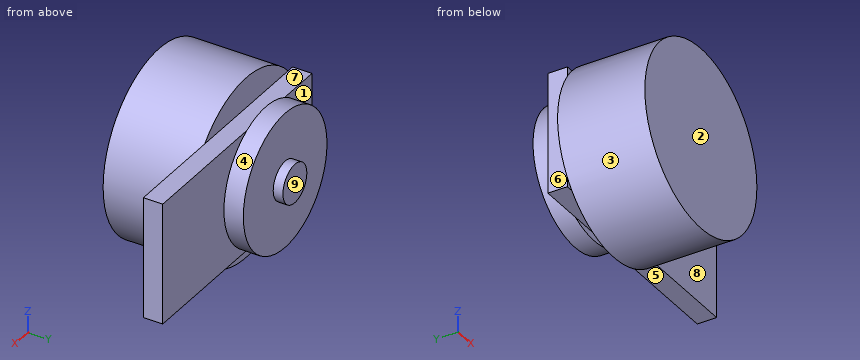
from build123d import *

# Parameters (mm, degrees)
SKETCH1_W           = 50
SKETCH1_H           = 25
BOSS_EXTRUDE1_DEPTH = 4
SKETCH2_R           = 14
BOSS_EXTRUDE2_DEPTH = 4
SKETCH3_R           = 4
BOSS_EXTRUDE3_DEPTH = 2
SKETCH4_R           = 18.75
BOSS_EXTRUDE4_DEPTH = 18


with BuildPart() as part:
    # Sketch1 → Boss-Extrude1 (new body)
    with BuildSketch(Plane(origin=(0, 0, 0), x_dir=(1, 0, 0), z_dir=(0, 1, 0))):
        Rectangle(SKETCH1_W, SKETCH1_H)
    extrude(amount=BOSS_EXTRUDE1_DEPTH)

    # Sketch2 → Boss-Extrude2 (add)
    with BuildSketch(Plane(origin=(0, 4, 0), x_dir=(1, 0, 0), z_dir=(0, 1, 0))):
        with Locations((-9.5, 0)):
            Circle(SKETCH2_R)
    extrude(amount=BOSS_EXTRUDE2_DEPTH)

    # Sketch3 → Boss-Extrude3 (add)
    with BuildSketch(Plane(origin=(0, 8, 0), x_dir=(1, 0, 0), z_dir=(0, 1, 0))):
        with Locations((-9.5, 0)):
            Circle(SKETCH3_R)
    extrude(amount=BOSS_EXTRUDE3_DEPTH)

    # Sketch4 → Boss-Extrude4 (add)
    with BuildSketch(Plane.XZ):
        with Locations((-9.5, 0)):
            Circle(SKETCH4_R)
    extrude(amount=BOSS_EXTRUDE4_DEPTH)


solid = part.part
Verification items for the finished model (mm, model axes). Face numbers are marked on the shaded views. A direction names the side the tool comes from. Round coordinates to 2 decimals unless told otherwise and drop trailing zeros. Loops run counter-clockwise (first coordinate to the right, second up) from the corner with the lowest first, then second, coordinate; pieces in that order, holes last. Notation, with made-up numbers: (86, -25.5) - (139, -25.5) arc R26 ccw to (139, -6.5) - close; hole circle Ø6 at (24, -30.5). An arc over 180 degrees is marked (long way). Use one line per item in the form item = value.
1. Access from +Z, -Z, +X, -X, +Y, -Y to the whole of each face (thin tool, end or side, straight path). Record for the marked faces 1, 2, 3, 4 and 5.
A:
face_1 = -X, +Y
face_2 = +Z, -Z, +X, -X, -Y
face_3 = -Y
face_4 = +Y
face_5 = -Z, +X, -X
2. Draft check along Y on the marked faces 6, 7, 8 and 9. Enter one of: pulls with the +Y half, pulls with the -Y half, needs draft (parallel to the pull), parting line crosses it, or undercut.
A:
face_6 = needs draft
face_7 = undercut
face_8 = pulls with the -Y half
face_9 = pulls with the +Y half
3. Section check B-B on x = -9.5. Record the cut outline in (y, z).
A:
outline = (-18, -18.75) - (0, -18.75) - (0, -12.5) - (4, -12.5) - (4, -14) - (8, -14) - (8, -4) - (10, -4) - (10, 4) - (8, 4) - (8, 14) - (4, 14) - (4, 12.5) - (0, 12.5) - (0, 18.75) - (-18, 18.75) - close
4. Section check D-D on x = 18. Record the cut outline in (y, z), and give its area (3 significant figures).
A:
outline = (0, -12.5) - (4, -12.5) - (4, 12.5) - (0, 12.5) - close
area = 100 mm²
5. Gauge pin test, flat ends, axial feed: pin 1 Ø7.5 at (x, z) = (-18.5, 5) entering from +Y; pin 2 Ø2 at (y, z) = (2, -10.5) entering from -X; pin 3 Ø6 at (x, y) = (13.5, -13) entering from +Z; pin 4 Ø12 at (y, z) = (-14.5, -9) entering from -X. Record the tip position at first contact, or that the pin passes through.
A:
pin_1 = 8
pin_2 = -25
pin_3 = through
pin_4 = -28.01
6. Scan lines: probe 1 along Y at (x, z) = (18.5, 8); probe 2 along Z at (x, y) = (-17, 2); probe 3 along Y at (x, z) = (-16.5, 15). Record each from-to range of solid material in increasing order.
A:
probe_1 = 0 to 4
probe_2 = -12.5 to 12.5
probe_3 = -18 to 0
7. Section check A-A on z = 0. Record the cut outline in (x, y).
A:
outline = (-28.25, -18) - (9.25, -18) - (9.25, 0) - (25, 0) - (25, 4) - (4.5, 4) - (4.5, 8) - (-5.5, 8) - (-5.5, 10) - (-13.5, 10) - (-13.5, 8) - (-23.5, 8) - (-23.5, 4) - (-25, 4) - (-25, 0) - (-28.25, 0) - close
8. Section check C-C on y = -10.75. Record the cut outline in (x, z).
A:
outline = circle Ø37.5 at (-9.5, 0)
